```python
from build123d import *

# Parameters (mm, degrees)
EXTRUDE_364_DEPTH   = 3
CUT_EXTRUDE_1_DEPTH = 44.269504273
CUT_EXTRUDE_2_DEPTH = 1
SKETCH_4_W          = 31
SKETCH_4_H          = 27
EXTRUDE_1_DEPTH     = 28
SKETCH_5_W          = 0.8
SKETCH_5_H          = 6.3
SKETCH_5_W_2        = 6.3
SKETCH_5_H_2        = 0.8
EXTRUDE_2_DEPTH     = 11
SKETCH_6_W          = 5
SKETCH_6_H          = 1.6
EXTRUDE_3_DEPTH     = 0.6
SKETCH_7_W          = 5
SKETCH_7_H          = 1.6
EXTRUDE_4_DEPTH     = 0.6
SKETCH_8_R          = 1
EXTRUDE_5_DEPTH     = 1


with BuildPart() as part:
    # ｽｹｯﾁ1 → Extrude 364 (new body)
    with BuildSketch(Plane(origin=(0, 0, 0), x_dir=(1, 0, 0), z_dir=(0, 1, 0))):
        Polygon((-3, 4), (-3, -4), (3.5, -13.5), (34.5, -13.5), (41, -4), (41, 4), (34.5, 13.5), (3.5, 13.5), align=None)
    extrude(amount=EXTRUDE_364_DEPTH)

    # ｽｹｯﾁ2 → ｶｯﾄ - 押し出し1 (cut, through all)
    with BuildSketch(Plane(origin=(0, 3, 0), x_dir=(-1, 0, 0), z_dir=(0, 1, 0))):
        with BuildLine():
            Line((-41, 1.75), (-38, 1.75))
            ThreePointArc((-38, 1.75), (-36.25, 0), (-38, -1.75))
            Line((-38, -1.75), (-41, -1.75))
            Line((-41, -1.75), (-41, 1.75))
        make_face()
        with BuildLine():
            Line((3, 1.75), (0, 1.75))
            ThreePointArc((0, 1.75), (-1.75, 0), (0, -1.75))
            Line((0, -1.75), (3, -1.75))
            Line((3, -1.75), (3, 1.75))
        make_face()
    extrude(amount=-CUT_EXTRUDE_1_DEPTH, mode=Mode.SUBTRACT)

    # ｽｹｯﾁ3 → ｶｯﾄ - 押し出し2 (cut)
    with BuildSketch(Plane.XZ):
        Polygon((39, 3.75), (39, 6.923076923), (34.5, 13.5), (3.5, 13.5), (-1, 6.923076923), (-1, 3.75), (-0.747712751, 3.75), (4.554918828, 11.5), (33.445081172, 11.5), (38.747712751, 3.75), align=None)
        with BuildLine():
            Line((38, 3.75), (38.747712751, 3.75))
            Line((38.747712751, 3.75), (33.445081172, 11.5))
            Line((33.445081172, 11.5), (4.554918828, 11.5))
            Line((4.554918828, 11.5), (-0.747712751, 3.75))
            Line((-0.747712751, 3.75), (0, 3.75))
            ThreePointArc((0, 3.75), (3.75, 0), (0, -3.75))
            Line((0, -3.75), (-0.747712751, -3.75))
            Line((-0.747712751, -3.75), (4.554918828, -11.5))
            Line((4.554918828, -11.5), (33.445081172, -11.5))
            Line((33.445081172, -11.5), (38.747712751, -3.75))
            Line((38.747712751, -3.75), (38, -3.75))
            ThreePointArc((38, -3.75), (34.25, 0), (38, 3.75))
        make_face()
        Polygon((39, -3.75), (38.747712751, -3.75), (33.445081172, -11.5), (4.554918828, -11.5), (-0.747712751, -3.75), (-1, -3.75), (-1, -6.923076923), (3.5, -13.5), (34.5, -13.5), (39, -6.923076923), align=None)
    extrude(amount=-CUT_EXTRUDE_2_DEPTH, mode=Mode.SUBTRACT)

    # ｽｹｯﾁ4 → ﾎﾞｽ - 押し出し1 (add)
    with BuildSketch(Plane(origin=(0, 3, 0), x_dir=(-1, 0, 0), z_dir=(0, 1, 0))):
        with Locations((-19, 0)):
            Rectangle(SKETCH_4_W, SKETCH_4_H)
    extrude(amount=EXTRUDE_1_DEPTH)

    # ｽｹｯﾁ5 → ﾎﾞｽ - 押し出し2 (add)
    with BuildSketch(Plane(origin=(0, 31, 0), x_dir=(-1, 0, 0), z_dir=(0, 1, 0))):
        with Locations((-6.6, -7.7)):
            Rectangle(SKETCH_5_W, SKETCH_5_H)
        with Locations((-6.6, 7.7)):
            Rectangle(SKETCH_5_W, SKETCH_5_H)
        with Locations((-27.5, -8.15)):
            Rectangle(SKETCH_5_W_2, SKETCH_5_H_2)
        with Locations((-27.5, 8.15)):
            Rectangle(SKETCH_5_W_2, SKETCH_5_H_2)
    extrude(amount=EXTRUDE_2_DEPTH)

    # ｽｹｯﾁ6 → ﾎﾞｽ - 押し出し3 (add)
    with BuildSketch(Plane.XY.offset(13.5)):
        with Locations((28.1, 28.45)):
            Rectangle(SKETCH_6_W, SKETCH_6_H)
    extrude(amount=EXTRUDE_3_DEPTH)

    # ｽｹｯﾁ7 → ﾎﾞｽ - 押し出し4 (add)
    with BuildSketch(Plane(origin=(0, 0, -13.5), x_dir=(-1, 0, 0), z_dir=(0, 0, -1))):
        with Locations((-9.9, 28.45)):
            Rectangle(SKETCH_7_W, SKETCH_7_H)
    extrude(amount=EXTRUDE_4_DEPTH)

    # ｽｹｯﾁ8 → ﾎﾞｽ - 押し出し5 (add)
    with BuildSketch(Plane.XZ.offset(-1)):
        with Locations(Location((19, 11.5, 0), (0, 0, 270))):
            Circle(SKETCH_8_R)
        with Locations(Location((19, -11.5, 0), (0, 0, 270))):
            Circle(SKETCH_8_R)
        with Locations(Location((36, 8, 0), (0, 0, 270))):
            Circle(SKETCH_8_R)
        with Locations(Location((36, -8, 0), (0, 0, 270))):
            Circle(SKETCH_8_R)
        with Locations(Location((2, 8, 0), (0, 0, 270))):
            Circle(SKETCH_8_R)
        with Locations(Location((2, -8, 0), (0, 0, 270))):
            Circle(SKETCH_8_R)
    extrude(amount=EXTRUDE_5_DEPTH)


solid = part.part
```
The model under review builds one solid part; all positions refer to its coordinate system, in mm. A direction names the side the tool comes from. Give positions to 0.01 mm unless a question says otherwise; leave off trailing zeros. Write each loop counter-clockwise with the first axis right and the second up, starting at its lowest first coordinate (ties: lowest second). Pieces come first, ordered by that corner, then holes.
(1) To check wall thickness, follow L1, parallel to Y at x = 12, z = -10.25; L2, parallel to Z at x = 22, y = 22; L3, parallel to X at y = 38.5, z = -6.5. State the ranges of each line that lie inside material, in increasing order.
(2) The part is to be moulded in two halves that separate along Z. For faces 5 (the cylindrical face through (1.11, 0.51, -8.46)), 6 (the flat face through (36, 3, 0)), 7 (the flat face through (28, 36, 8.55)), say which applies: released by +Z, released by -Z, zero draft, split by the parting line, or undercut.
(3) Consider section C-C, the plane x = 4.5. Give the boundary of the cut face in (y, z), and give its area (3 significant figures).
(4) Tool access review of faces 1 (the flat face through (34.5, 17, 0)), 2 (the cylindrical face through (1.4, 0.5, 8.8)), 3 (the flat face through (28, 36, -7.75)), 4 (the flat face through (6.2, 36, -8)): name each direction out of +Z, -Z, +X, -X, +Y, -Y from which nothing blocks a thin tool from reaching the whole face with its end or side.
(5) Consider section B-B, the plane z = 0. Give the boundary of the cut face in (x, y).
(6) Consider section A-A, the plane y = 33.5. Give the boundary of the cut face in (x, z), and give its area (3 significant figures).
(7) Consider section D-D, the plane y = 20. Give the boundary of the cut face in (x, z), and give its area (3 significant figures).
(8) For P1, Ø5, axis at x = 35.5, y = 7, coming from the +Z side; P2, Ø3, axis at y = 14, z = 6, coming from the +X side; P3, Ø7, axis at x = 36.5, z = -1.5, coming from the +Y side, all flat-tipped, find the tip position at first contact; note any pin that passes through.
Returned:
1. L1: y = 1 to 31
1. L2: z = -13.5 to 13.5
1. L3: x = 6.2 to 7
2. face 5: undercut
2. face 6: zero draft
2. face 7: released by +Z
3. outline: (1, -13.5) - (31, -13.5) - (31, 13.5) - (1, 13.5) - close
3. area: 810 mm2
4. face 1: +Z, -Z, +X, +Y
4. face 2: -Y
4. face 3: +X, +Y
4. face 4: +Z, -Z, -X, +Y
5. outline: (1.75, 0) - (3.75, 0) - (3.75, 1) - (34.25, 1) - (34.25, 0) - (36.25, 0) - (36.25, 3) - (34.5, 3) - (34.5, 31) - (3.5, 31) - (3.5, 3) - (1.75, 3) - close
6. outline: (6.2, -10.85) - (7, -10.85) - (7, -4.55) - (6.2, -4.55) - close; (6.2, 4.55) - (7, 4.55) - (7, 10.85) - (6.2, 10.85) - close; (24.35, -8.55) - (30.65, -8.55) - (30.65, -7.75) - (24.35, -7.75) - close; (24.35, 7.75) - (30.65, 7.75) - (30.65, 8.55) - (24.35, 8.55) - close
6. area: 20.2 mm2
7. outline: (3.5, -13.5) - (34.5, -13.5) - (34.5, 13.5) - (3.5, 13.5) - close
7. area: 837 mm2
8. P1: stops at z = 13.5
8. P2: stops at x = 34.5
8. P3: stops at y = 31
